Job drawing, mm, ordinate dimensions from the low corner. One solid piece. Round coordinates to 2 decimals unless told otherwise and drop trailing zeros. Loops run counter-clockwise (first coordinate to the right, second up) from the corner with the lowest first, then second, coordinate; pieces in that order, holes last.
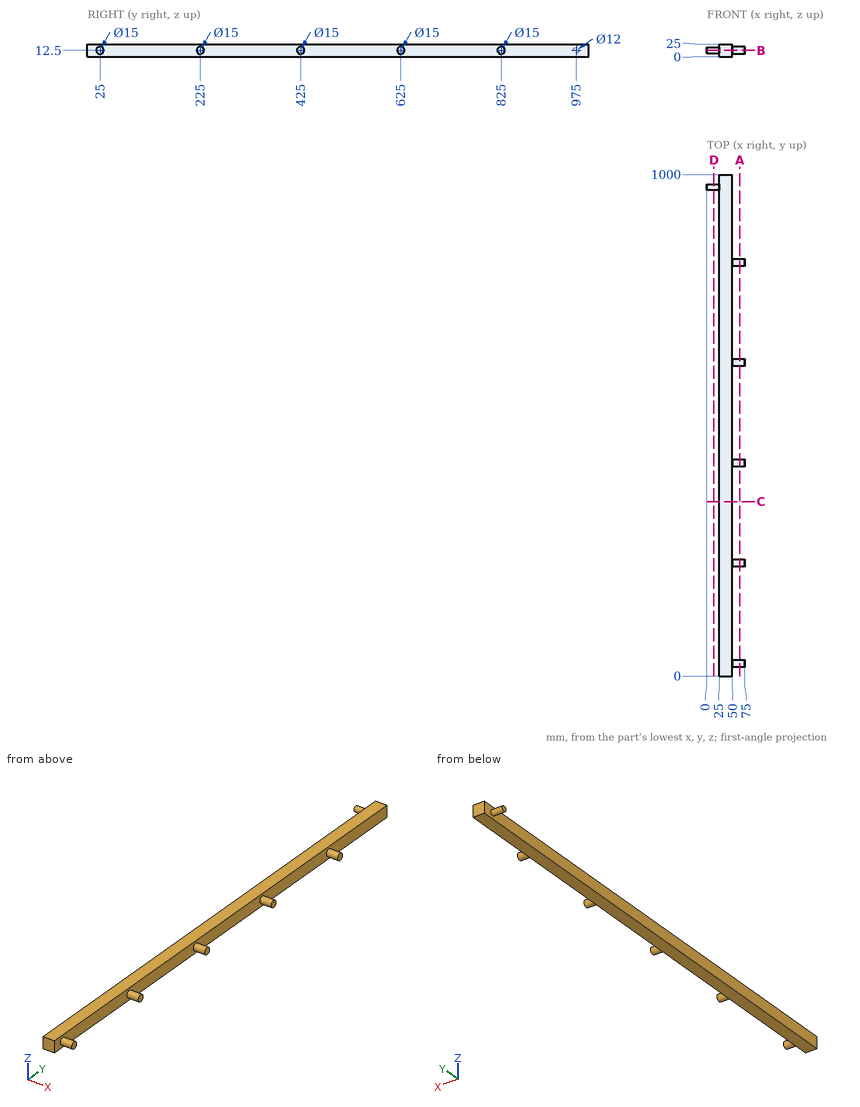
Item 1: Cut at B-B, the plane z = 12.5. Give the cut face in (x, y), plus the area to 3 significant figures.
Answers follow:
outline: (0, 969) - (25, 969) - (25, 0) - (50, 0) - (50, 17.5) - (75, 17.5) - (75, 32.5) - (50, 32.5) - (50, 217.5) - (75, 217.5) - (75, 232.5) - (50, 232.5) - (50, 417.5) - (75, 417.5) - (75, 432.5) - (50, 432.5) - (50, 617.5) - (75, 617.5) - (75, 632.5) - (50, 632.5) - (50, 817.5) - (75, 817.5) - (75, 832.5) - (50, 832.5) - (50, 1000) - (25, 1000) - (25, 981) - (0, 981) - close
area: 27,200 mm2
Item 2: Cut at A-A, the plane x = 65.5. Give the cut face in (y, z).
Answers follow:
outline: circle Ø15 at (25, 12.5); circle Ø15 at (225, 12.5); circle Ø15 at (425, 12.5); circle Ø15 at (625, 12.5); circle Ø15 at (825, 12.5)
Item 3: Probe line 1 (Y direction, x = 57, z = 12.75); line 2 (Y direction, x = 51.5, z = 6.75); line 3 (X direction, y = 137, z = 18.5). List the from-to ranges inside material, lowest first.
Answers follow:
line 1: y = 17.5 to 32.5, 217.5 to 232.5, 417.5 to 432.5, 617.5 to 632.5, 817.5 to 832.5
line 2: y = 20.18 to 29.82, 220.18 to 229.82, 420.18 to 429.82, 620.18 to 629.82, 820.18 to 829.82
line 3: x = 25 to 50
Item 4: Cut at C-C, the plane y = 347.5. Give the cut face in (x, z), plus the area to 3 significant figures.
Answers follow:
outline: (25, 0) - (50, 0) - (50, 25) - (25, 25) - close
area: 625 mm2
Item 5: Flat gauge pins, fed straight in: P1, Ø1, axis at y = 503, z = 17.5, coming from the +X side; P2, Ø12.5, axis at y = 667.5, z = 8.5, coming from the -X side; P3, Ø2, axis at x = 60.5, z = 8, coming from the +Y side. Where does each tip first touch, or does it go through?
Answers follow:
P1: stops at x = 50
P2: stops at x = 25
P3: stops at y = 831.63
Item 6: Cut at D-D, the plane x = 14. Give the cut face in (y, z), plus the area to 3 significant figures.
Answers follow:
outline: circle Ø12 at (975, 12.5)
area: 113 mm2
